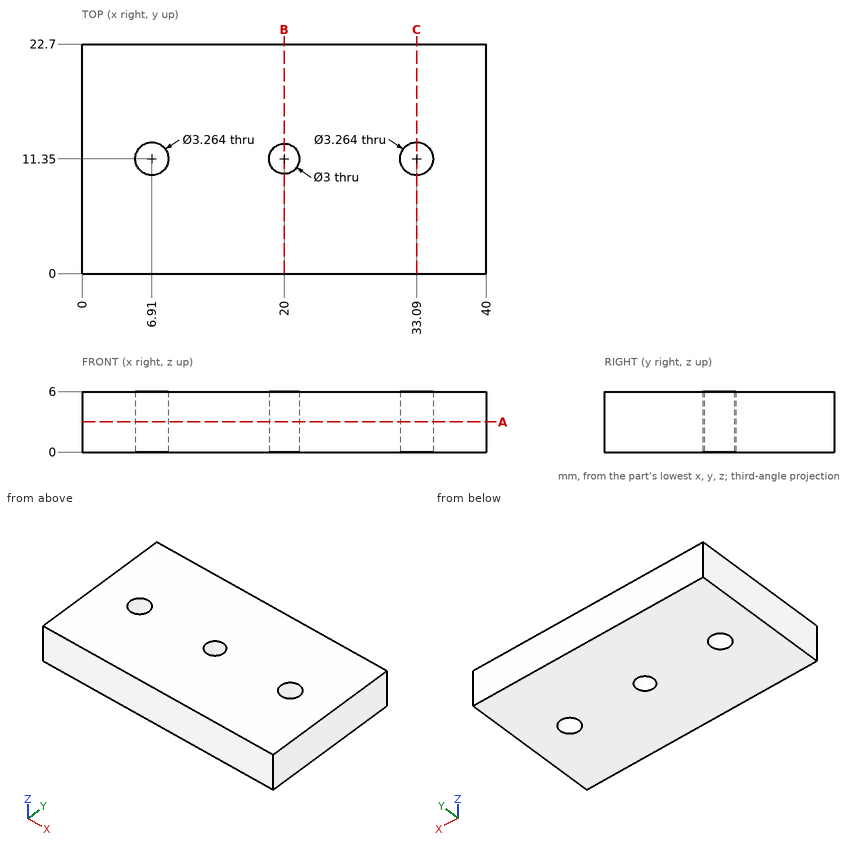
Answer from the drawing. Dimensions are ordinates in mm from the lowest x, y and z of the part. Coordinates: 2 decimals unless noted, no trailing zeros. Loops run counter-clockwise (first coordinate to the right, second up) from the corner with the lowest first, then second, coordinate; pieces in that order, holes last.
1) Section B-B (x = 20) is taken. Give the vertices of the cut face in (y, z), plus the area to 3 significant figures.
Results:
outline: (0, 0) - (9.85, 0) - (9.85, 6) - (0, 6) - close; (12.85, 0) - (22.7, 0) - (22.7, 6) - (12.85, 6) - close
area: 118 mm2
2) Section C-C (x = 33.09) is taken. Give the vertices of the cut face in (y, z).
Results:
outline: (0, 0) - (9.72, 0) - (9.72, 6) - (0, 6) - close; (12.98, 0) - (22.7, 0) - (22.7, 6) - (12.98, 6) - close
3) Section A-A (z = 3) is taken. Give the vertices of the cut face in (x, y).
Results:
outline: (0, 0) - (40, 0) - (40, 22.7) - (0, 22.7) - close; hole circle Ø3.26 at (6.91, 11.35); hole circle Ø3 at (20, 11.35); hole circle Ø3.26 at (33.09, 11.35)
4) Consider probe 1 along Y at (x, z) = (33.09, 3.8); probe 2 along X at (y, z) = (10.5, 3.35). Determine where each line is inside the solid, lowest interval first.
Results:
probe 1: y = 0 to 9.72, 12.98 to 22.7
probe 2: x = 0 to 5.52, 8.3 to 18.76, 21.24 to 31.7, 34.48 to 40
